```python
from build123d import *

# Parameters (mm, degrees)
SKETCH_1_W          = 25
SKETCH_1_H          = 45
EXTRUDE_1_DEPTH     = 110
SKETCH_2_W          = 15
SKETCH_2_H          = 15
CUT_EXTRUDE_2_DEPTH = 110
SKETCH_3_W          = 35
SKETCH_3_H          = 15
CUT_EXTRUDE_3_DEPTH = 38
SKETCH_4_W          = 7
SKETCH_4_H          = 60
CUT_EXTRUDE_4_DEPTH = 38
SKETCH_5_W          = 35
SKETCH_5_H          = 15
CUT_EXTRUDE_5_DEPTH = 38
FILLET_1_R          = 5
SKETCH_6_W          = 7
SKETCH_6_H          = 60
CUT_EXTRUDE_6_DEPTH = 38
FILLET_3_R          = 5
SKETCH_7_R          = 2.5
CUT_EXTRUDE_7_DEPTH = 40


with BuildPart() as part:
    # 草图1 → 凸台-拉伸1 (new body)
    with BuildSketch(Plane(origin=(0, 0, 0), x_dir=(1, 0, 0), z_dir=(0, 1, 0))):
        Rectangle(SKETCH_1_W, SKETCH_1_H)
    extrude(amount=EXTRUDE_1_DEPTH)

    # 草图2 → 切除-拉伸2 (cut)
    with BuildSketch(Plane(origin=(0, 110, 0), x_dir=(1, 0, 0), z_dir=(0, 1, 0))):
        with Locations((-5, 0)):
            Rectangle(SKETCH_2_W, SKETCH_2_H)
    extrude(amount=-CUT_EXTRUDE_2_DEPTH, mode=Mode.SUBTRACT)

    # 草图3 → 切除-拉伸3 (cut)
    with BuildSketch(Plane.ZY.offset(12.5)):
        with Locations((0, 12.5)):
            Rectangle(SKETCH_3_W, SKETCH_3_H)
    extrude(amount=-CUT_EXTRUDE_3_DEPTH, mode=Mode.SUBTRACT)

    # 草图4 → 切除-拉伸4 (cut)
    with BuildSketch(Plane.ZY.offset(12.5)):
        with Locations((19, 55)):
            Rectangle(SKETCH_4_W, SKETCH_4_H)
    extrude(amount=-CUT_EXTRUDE_4_DEPTH, mode=Mode.SUBTRACT)

    # 草图5 → 切除-拉伸5 (cut)
    with BuildSketch(Plane.ZY.offset(12.5)):
        with Locations((0, 97.5)):
            Rectangle(SKETCH_5_W, SKETCH_5_H)
    extrude(amount=-CUT_EXTRUDE_5_DEPTH, mode=Mode.SUBTRACT)

    # 圆角1
    fillet_1_edges = [part.edges().sort_by_distance(p)[0] for p in [
        (0, 25, 15.5),
        (0, 85, 15.5),
    ]]
    fillet(fillet_1_edges, radius=FILLET_1_R)

    # 草图6 → 切除-拉伸6 (cut)
    with BuildSketch(Plane.ZY.offset(12.5)):
        with Locations((-19, 57.659101088)):
            Rectangle(SKETCH_6_W, SKETCH_6_H)
    extrude(amount=-CUT_EXTRUDE_6_DEPTH, mode=Mode.SUBTRACT)

    # 圆角3
    fillet_3_edges = [part.edges().sort_by_distance(p)[0] for p in [
        (0, 87.659101088, -15.5),
        (0, 27.659101088, -15.5),
    ]]
    fillet(fillet_3_edges, radius=FILLET_3_R)

    # 草图7 → 切除-拉伸7 (cut)
    with BuildSketch(Plane(origin=(0, 0, -15.5), x_dir=(-1, 0, 0), z_dir=(0, 0, -1))):
        with Locations((5, 40)):
            Circle(SKETCH_7_R)
        with Locations((5, 70)):
            Circle(SKETCH_7_R)
    extrude(amount=-CUT_EXTRUDE_7_DEPTH, mode=Mode.SUBTRACT)


solid = part.part
```
Part model, mm, in its own coordinate system. A direction names the side the tool comes from. Round coordinates to 2 decimals unless told otherwise and drop trailing zeros. Write each loop counter-clockwise with the first axis right and the second up, starting at its lowest first coordinate (ties: lowest second). Pieces come first, ordered by that corner, then holes. Notation, with made-up numbers: (29.25, 4.25) -> (78.25, 4.25) arc R21 cw to (78.25, 38.25) -> close; hole circle Ø6 at (34.5, 62). An arc over 180 degrees is marked (long way). Return JSON: item names as keys, results as strings. Group by question number.
Q1. Saw through at B-B on y = 70. Write the cut outline in (x, z), plus the area to 3 significant figures.
Q2. Probe L1, parallel to Y at x = -5, z = 10.75; L2, parallel to Y at x = 3.5, z = 14.5; L3, parallel to Z at x = -3.25, y = 8. List the from-to ranges inside material, lowest first. Write a range as [from, to].
Q3. Pin check, flat tips, straight feed: pin 1 (8 mm diameter, centred on x = -5, y = 40, fed in from +Z); pin 2 (4 mm diameter, centred on y = 3.5, z = -2, fed in from -X); pin 3 (7.5 mm diameter, centred on x = -6, y = 46, fed in from -Z). Stop position of each tip, or through.
Q4. Mould opens along Y. For faces 5 (the flat face through (0, 12, 22.5)), 6 (the flat face through (0, 57, -15.5)), 7 (the flat face through (3, 110, 0)) say: pulls with the +Y half, pulls with the -Y half, needs draft (parallel to the pull), parting line crosses it, or undercut.
Q5. Saw through at A-A on z = 5.5. Write the cut outline in (x, y).
Q6. Saw through at D-D on y = 58. Write the cut outline in (x, z).
Q7. Which spindle directions (+Z, -Z, +X, -X, +Y, -Y) get a long thin tool onto all of the face, cutting with end or side? Do faces 1 (the flat face through (0, 25, 21)), 2 (the cylindrical face through (0.175, 29.085, -17.004)), 3 (the flat face through (-5, 108, -7.5)), 4 (the flat face through (3, 90, 0)). Say none if no direction does.
Q8. Saw through at C-C on x = -5. State how many separate pieces and enclosed holes the cut face has, plus the area to 3 significant figures.
Answer:
{
 "1": {"outline": "(-12.5, -15.5) -> (-7.5, -15.5) -> (-7.5, -7.5) -> (-12.5, -7.5) -> close; (-12.5, 7.5) -> (-7.5, 7.5) -> (-7.5, 15.5) -> (-12.5, 15.5) -> close; (-2.5, -15.5) -> (12.5, -15.5) -> (12.5, 15.5) -> (-2.5, 15.5) -> (-2.5, 7.5) -> (2.5, 7.5) -> (2.5, -7.5) -> (-2.5, -7.5) -> close", "area": "470 mm2"},
 "2": {"L1": "[0, 5], [20, 37.5], [42.5, 67.5], [72.5, 90], [105, 110]", "L2": "[0, 5], [20, 90], [105, 110]", "L3": "[-22.5, -17.5], [17.5, 22.5]"},
 "3": {"pin 1": "z = 15.5", "pin 2": "x = 2.5", "pin 3": "z = -15.5"},
 "4": {"face 5": "needs draft", "face 6": "undercut", "face 7": "pulls with the +Y half"},
 "5": {"outline": "(2.5, 0) -> (12.5, 0) -> (12.5, 5) -> (2.5, 5) -> close; (2.5, 20) -> (12.5, 20) -> (12.5, 90) -> (2.5, 90) -> close; (2.5, 105) -> (12.5, 105) -> (12.5, 110) -> (2.5, 110) -> close"},
 "6": {"outline": "(-12.5, -15.5) -> (12.5, -15.5) -> (12.5, 15.5) -> (-12.5, 15.5) -> (-12.5, 7.5) -> (2.5, 7.5) -> (2.5, -7.5) -> (-12.5, -7.5) -> close"},
 "7": {"face 1": "+Z, +X, -X", "face 2": "-Z, +X, -X", "face 3": "-X, +Y, -Y", "face 4": "+X, -X"},
 "8": {"separate pieces": "6", "enclosed holes": "0", "area": "1,720 mm2"}
}
